Verification items for the finished model (mm, model axes). A direction names the side the tool comes from. Coordinates: 2 decimals unless noted, no trailing zeros. Order: outer loops, then holes, each group sorted by start corner. A loop starts at its lowest first (then second) coordinate and runs counter-clockwise, first axis right, second up. Notation, with made-up numbers: M 22,-39 L 39,-39 A24 ccw 39,-21 Z; hole C 89,-33 d5. An arc over 180 degrees is marked long. Answer as a JSON object with one key per item and string values. Group by question number.
(1) Material ranges on line 1 (X direction, y = 0.5, z = -523); line 2 (Y direction, x = -7, z = -134.5), recorded low to high.
(2) Cross-section at B-B (z = -387). Enter the section's corners in (x, y).
(3) Mould release check, pull along X, two halves, no side actions. Record for faces 3 (the face through (89.874, -68.913, 60.829)), 4 (the face through (9.104, -40.997, 1.622)), 5 (the face through (96, -61, 84.203)): released by +X, released by -X, zero draft, split by the parting line, or undercut.
(4) Cross-section at A-A (y = 0). Enter the section's corners in (x, z).
(5) Access from +Z, -Z, +X, -X, +Y, -Y to the whole of each face (thin tool, end or side, straight path). Record for faces 1 (the face through (-36.34, 11.44, -579.5)), 2 (the face through (-31.5, 9.9, -561.8)).
(6) Gauge pin test, flat ends, axial feed: pin 1 Ø1.5 at (y, z) = (-7, -326.5) entering from -X; pin 2 Ø8 at (x, y) = (73.5, 85.5) entering from -Z; pin 3 Ø1.6 at (y, z) = (33.5, -1099.5) entering from +X. Record the tip position at first contact, or that the pin passes through.
from build123d import *

# Parameters (mm, degrees)
F3_DEPTH = 63.5


with BuildPart() as f1:
    # F0 (on Front) → F1 (revolve)
    with BuildSketch(Plane.XZ):
        Polygon((-113.253824, 36.790495), (-113.253824, 84.202737), (-118.333824, 84.202737), (-118.333824, 33.402737), (-38.1, 0), (-38.1, -1143), (-33.02, -1143), (-33.02, 3.387759), align=None)
    revolve(axis=Axis((0, 0, -529.398632), (0, 0, -1)))

    # F2 (on Front) → F3 (cut, symmetric)
    with BuildSketch(Plane.XZ):
        with BuildLine():
            Line((8.060034, -1012.105305), (8.060034, -1153.510451))
            Line((8.060034, -1153.510451), (58.457147, -1153.510451))
            Line((58.457147, -1153.510451), (58.457147, -966.385305))
            Line((58.457147, -966.385305), (53.780034, -966.385305))
            ThreePointArc((53.780034, -966.385305), (21.451112, -979.776383), (8.060034, -1012.105305))
        make_face()
    extrude(amount=F3_DEPTH, both=True, mode=Mode.SUBTRACT)


solid = f1.part
Taken from the geometry:
{
 "1": {"line 1": "x = -38.1 to -33.02, 33.02 to 38.1", "line 2": "y = -37.45 to -32.27, 32.27 to 37.45"},
 "2": {"outline": "C 0,0 d76.2; hole C 0,0 d66.04"},
 "3": {"face 3": "undercut", "face 4": "split by the parting line", "face 5": "zero draft"},
 "4": {"outline": "M -118.33,33.4 L -38.1,0 L -38.1,-1143 L -33.02,-1143 L -33.02,3.39 L -113.25,36.79 L -113.25,84.2 L -118.33,84.2 Z; M 33.02,-971.37 A45.72 cw 38.1,-969.16 L 38.1,0 L 118.33,33.4 L 118.33,84.2 L 113.25,84.2 L 113.25,36.79 L 33.02,3.39 Z"},
 "5": {"face 1": "-Z", "face 2": "+Z, -Z"},
 "6": {"pin 1": "stops at x = -37.58", "pin 2": "stops at z = 29.41", "pin 3": "stops at x = 8.06"}
}
